Could you check a few things on this drawing? It's one solid part, dimensions in mm from its lowest x, y, z. Round coordinates to 2 decimals unless told otherwise and drop trailing zeros. Write each loop counter-clockwise with the first axis right and the second up, starting at its lowest first coordinate (ties: lowest second). Pieces come first, ordered by that corner, then holes. Notation, with made-up numbers: (57, -1) -> (115, -1) arc R22 cw to (115, 38) -> close; hole circle Ø3 at (58, 64). An arc over 180 degrees is marked (long way). Answer in a Markdown table with one row per item.
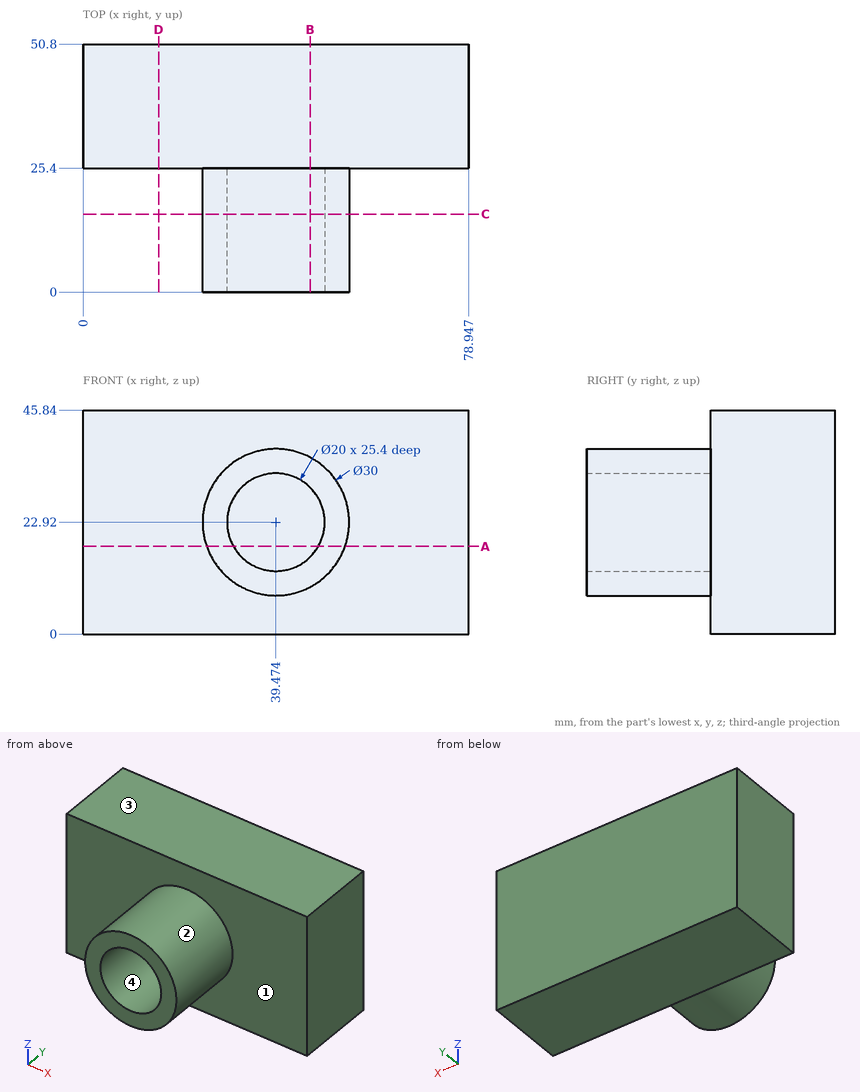
1) Imagine slicing it at D-D, the plane x = 15.5. Please give me the cut outline in (y, z).
Findings:
| item | result |
|---|---|
| outline | (25.4, 0) -> (50.8, 0) -> (50.8, 45.84) -> (25.4, 45.84) -> close |
2) Imagine slicing it at B-B, the plane x = 46.5. Please give me the cut outline in (y, z) (1 decimal).
Findings:
| item | result |
|---|---|
| outline | (0, 9.7) -> (25.4, 9.7) -> (25.4, 0) -> (50.8, 0) -> (50.8, 45.8) -> (25.4, 45.8) -> (25.4, 36.2) -> (0, 36.2) -> (0, 30) -> (25.4, 30) -> (25.4, 15.8) -> (0, 15.8) -> close |
3) Thinking about a two-plate mould opening in Z: for the marked faces 1, 2, 3 and 4, which applies, +Z half, -Z half, draft (parallel to the pull), parting line (faces both ways), or undercut?
Findings:
| item | result |
|---|---|
| face 1 | draft |
| face 2 | parting line |
| face 3 | +Z half |
| face 4 | undercut |
4) For pin 1 (5 mm diameter, centred on x = 70.5, z = 35, fed in from -Y); pin 2 (22 mm diameter, centred on x = 42.5, z = 21, fed in from -Y), each with a flat end and sliding along its axis, tell me the tip position at first contact or that it passes through.
Findings:
| item | result |
|---|---|
| pin 1 | stops at y = 25.4 |
| pin 2 | stops at y = 0 |
5) Please list where these lines run through material, in increasing order: line 1 (Y direction, x = 40.5, z = 3.5); line 2 (X direction, y = 3, z = 26) (1 decimal); line 3 (X direction, y = 3, z = 26.5) (1 decimal).
Findings:
| item | result |
|---|---|
| line 1 | y = 25.4 to 50.8 |
| line 2 | x = 24.8 to 30, 49 to 54.2 |
| line 3 | x = 24.9 to 30.1, 48.8 to 54 |
6) Imagine slicing it at C-C, the plane y = 16. Please give me the cut outline in (x, z).
Findings:
| item | result |
|---|---|
| outline | circle Ø30 at (39.47, 22.92); hole circle Ø20 at (39.47, 22.92) |
7) Imagine slicing it at A-A, the plane z = 18. Please give me the cut outline in (x, y), plus the area to 3 significant figures.
Findings:
| item | result |
|---|---|
| outline | (0, 25.4) -> (25.3, 25.4) -> (25.3, 0) -> (30.77, 0) -> (30.77, 25.4) -> (48.18, 25.4) -> (48.18, 0) -> (53.64, 0) -> (53.64, 25.4) -> (78.95, 25.4) -> (78.95, 50.8) -> (0, 50.8) -> close |
| area | 2,280 mm^2 |
